Build history of the part. All positions in model axes, mm. A direction names the side the tool comes from. Round coordinates to 2 decimals unless told otherwise and drop trailing zeros. Write each loop counter-clockwise with the first axis right and the second up, starting at its lowest first coordinate (ties: lowest second). Pieces come first, ordered by that corner, then holes.
Item 1: Mould opens along X. For faces 1 (the flat face through (0, -5, 53)), 2 (the flat face through (-20.787, -3.254, 21.154)), 3 (the cylindrical face through (3.94, -0.86, 56.1)), 4 (the cylindrical face through (-35.18, -3.25, 49.82)) say: +X half, -X half, draft (parallel to the pull), parting line (faces both ways), or undercut.
Item 2: 3-axis set-ups, long thin cutter, end or side, ignore diameter. For faces 5 (the cylindrical face through (4.056, -3.221, 3.685)), 6 (the cylindrical face through (3.94, -5.74, 56.1)), 7 (the flat face through (-13, -3, 47)): which of +Z, -Z, +X, -X, +Y, -Y reach the whole face in a straight line?
Item 3: Band-saw the part on C-C, the plane z = 4.5. Write the cut outline in (x, y), then the cut area to 3 significant figures.
Item 4: Wall check: probe 1 along Z at (x, y) = (-36, -1.75); probe 2 along Z at (x, y) = (-26, -4.75); probe 3 along Z at (x, y) = (-36.5, -5.5). Give the ranges that are in metal, low to high.
Item 5: Band-saw the part on B-B, the plane x = -36. Write the cut outline in (y, z).
Item 6: Band-saw the part on A-A, the plane z = 41. Write the cut outline in (x, y).
Item 7: Band-saw the part on D-D, the plane z = 21. Write the cut outline in (x, y).
Item 8: Drop flat-ended pins along their axis: pin 1 Ø2 at (x, y) = (-19, -4.5) entering from +Z; pin 2 Ø3.5 at (y, z) = (-3.5, 6.5) entering from -X. Give the stop position or say it passes through.
```python
from build123d import *

# Parameters (mm, degrees)
F0_R     = 1.778
F1_DEPTH = 6.6
F3_DEPTH = 8
F4_R     = 3


with BuildPart() as f1:
    # F0 (on Front) → F1 (new body)
    with BuildSketch(Plane.XZ):
        with BuildLine():
            Line((0, 10), (0, 0))
            Line((0, 0), (8, 0))
            Line((8, 0), (8, 27))
            ThreePointArc((8, 27), (5, 32), (8, 37))
            Line((8, 37), (8, 57))
            Line((8, 57), (0, 57))
            Line((0, 57), (0, 47))
            Line((0, 47), (-26, 47))
            ThreePointArc((-26, 47), (-29.535534, 48.464466), (-31, 52))
            Line((-31, 52), (-31, 67))
            Line((-31, 67), (-41, 67))
            Line((-41, 67), (-41, 32))
            Line((-41, 32), (0, 10))
        make_face()
        with Locations((-26, 41)):
            Circle(F0_R, mode=Mode.SUBTRACT)
        with Locations((-36, 51.396919)):
            Circle(F0_R, mode=Mode.SUBTRACT)
        with Locations((-36, 61.396919)):
            Circle(F0_R, mode=Mode.SUBTRACT)
    extrude(amount=F1_DEPTH)

    # F2 (on face) → F3 (cut, through all)
    with BuildSketch(Plane.YZ.offset(8)):
        with BuildLine():
            Line((-1.543041, 50.86), (-1.543041, 51.894725))
            ThreePointArc((-1.543041, 51.894725), (-3.436768, 53.394732), (-5.078, 51.622))
            Line((-5.078, 51.622), (-5.078, 50.587275))
            ThreePointArc((-5.078, 50.587275), (-3.184273, 49.087268), (-1.543041, 50.86))
        make_face()
        with BuildLine():
            ThreePointArc((-5.078, 5.187275), (-3.184273, 3.687268), (-1.543041, 5.46))
            Line((-1.543041, 5.46), (-1.543041, 6.494725))
            ThreePointArc((-1.543041, 6.494725), (-3.436768, 7.994732), (-5.078, 6.222))
            Line((-5.078, 6.222), (-5.078, 5.187275))
        make_face()
    extrude(amount=-F3_DEPTH, mode=Mode.SUBTRACT)

    # F4
    f4_edges = [f1.edges().sort_by_distance(p)[0] for p in [
        (4, 0, 57),
        (4, -6.6, 57),
    ]]
    fillet(f4_edges, radius=F4_R)


solid = f1.part
```
Results:
1. face 1: undercut
1. face 2: -X half
1. face 3: draft
1. face 4: undercut
2. face 5: +X, -X
2. face 6: +Z, +X, -Y
2. face 7: +Z, +Y, -Y
3. outline: (0, -6.6) - (8, -6.6) - (8, -4.82) - (0, -4.82) - close; (0, -1.82) - (8, -1.82) - (8, 0) - (0, 0) - close
3. area: 28.9 mm2
4. probe 1: z = 29.32 to 49.62, 53.17 to 59.62, 63.17 to 67
4. probe 2: z = 23.95 to 39.22, 42.78 to 47
4. probe 3: z = 29.59 to 49.69, 53.1 to 59.69, 63.1 to 67
5. outline: (-6.6, 29.32) - (0, 29.32) - (0, 49.62) - (-6.6, 49.62) - close; (-6.6, 53.17) - (0, 53.17) - (0, 59.62) - (-6.6, 59.62) - close; (-6.6, 63.17) - (0, 63.17) - (0, 67) - (-6.6, 67) - close
6. outline: (-41, -6.6) - (-27.78, -6.6) - (-27.78, 0) - (-41, 0) - close; (-24.22, -6.6) - (8, -6.6) - (8, 0) - (-24.22, 0) - close
7. outline: (-20.5, -6.6) - (8, -6.6) - (8, 0) - (-20.5, 0) - close
8. pin 1: stops at z = 47
8. pin 2: stops at x = 0
